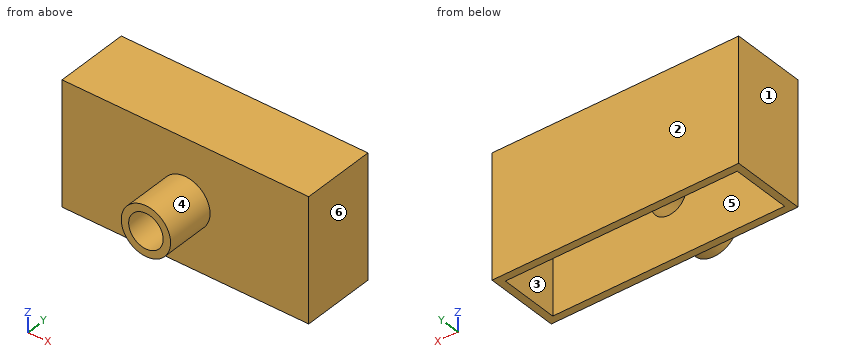
```python
from build123d import *

# Parameters (mm, degrees)
F0_W     = 254
F0_H     = 127
F1_DEPTH = 76.2
F2_W     = 25.4
F2_H     = 50.8
F4_T     = -7.62


with BuildPart() as f1:
    # F0 (on Front) → F1 (new body)
    with BuildSketch(Plane.XZ):
        Rectangle(F0_W, F0_H)
    extrude(amount=F1_DEPTH)

    # F2 (on Top) → F3 (revolve)
    with BuildSketch(Plane.XY):
        with Locations((12.7, -101.6)):
            Rectangle(F2_W, F2_H)
    revolve(axis=Axis((0, -101.6, 0), (0, 1, 0)))

    # F4
    f4_openings = [f1.faces().sort_by_distance(p)[0] for p in [
        (0, -127, 0),
        (0, -38.1, -63.5),
    ]]
    offset(amount=F4_T, openings=f4_openings, kind=Kind.INTERSECTION)


solid = f1.part
```
Source: CAD feature listing. Evaluate the final solid. Frame: model axes, mm. Face numbers are marked on the shaded views. A direction names the side the tool comes from. Coordinates: 2 decimals unless noted, no trailing zeros. Loops run counter-clockwise (first coordinate to the right, second up) from the corner with the lowest first, then second, coordinate; pieces in that order, holes last. Notation, with made-up numbers: (48.5, 84.25) -> (74.5, 84.25) arc R20 cw to (74.5, 122.25) -> close; hole circle Ø2 at (31, 20). An arc over 180 degrees is marked (long way). One line per item, written item: value. Start each with the question number.
Q1. Section query C-C, the plane y = -59. Return the cut outline in (x, z).
Q2. Section query D-D, the plane x = 75. Return the cut outline in (y, z).
Q3. Contact query for flat-ended pins moving along their axis: P1, Ø21.5, axis at x = 0, z = 0, coming from the -Y side; P2, Ø10, axis at x = -22, y = -28.5, coming from the -Z side. Output: stop coordinate, or through.
Q4. Section query A-A, the plane z = 48. Return the cut outline in (x, y), and give its area (3 significant figures).
Q5. Mould query, pull axis Y, two halves, no side actions, for the marked faces 1, 2 and 3. Classes: pulls with the +Y half, pulls with the -Y half, needs draft (parallel to the pull), parting line crosses it, or undercut.
Q6. Section query B-B, the plane x = 0. Return the cut outline in (y, z).
Q7. Set-up query: the marked faces 4, 5 and 6. Return all of +Z, -Z, +X, -X, +Y, -Y with unobstructed straight access to the full face (end or side cutting, diameter ignored); none if empty.
Q8. Line query: line 1 along Y through (x, z) = (79, 15.5); line 2 along X through (y, z) = (-107.5, 0); line 3 along X through (y, z) = (-36, 40.5). Output: solid intervals per line, ascending.
Results:
1. outline: (-127, -63.5) -> (-119.38, -63.5) -> (-119.38, 55.88) -> (119.38, 55.88) -> (119.38, -63.5) -> (127, -63.5) -> (127, 63.5) -> (-127, 63.5) -> close
2. outline: (-76.2, -63.5) -> (-68.58, -63.5) -> (-68.58, 55.88) -> (-7.62, 55.88) -> (-7.62, -63.5) -> (0, -63.5) -> (0, 63.5) -> (-76.2, 63.5) -> close
3. P1: y = -7.62
3. P2: z = 55.88
4. outline: (-127, -76.2) -> (127, -76.2) -> (127, 0) -> (-127, 0) -> close; hole (-119.38, -68.58) -> (119.38, -68.58) -> (119.38, -7.62) -> (-119.38, -7.62) -> close
4. area: 4,800 mm^2
5. face 1: needs draft
5. face 2: pulls with the +Y half
5. face 3: undercut
6. outline: (-127, -25.4) -> (-76.2, -25.4) -> (-76.2, -63.5) -> (-68.58, -63.5) -> (-68.58, -17.78) -> (-127, -17.78) -> close; (-127, 17.78) -> (-68.58, 17.78) -> (-68.58, 55.88) -> (-7.62, 55.88) -> (-7.62, -63.5) -> (0, -63.5) -> (0, 63.5) -> (-76.2, 63.5) -> (-76.2, 25.4) -> (-127, 25.4) -> close
7. face 4: -Y
7. face 5: -Z
7. face 6: +Z, -Z, +X, +Y, -Y
8. line 1: -76.2 to -68.58, -7.62 to 0
8. line 2: -25.4 to -17.78, 17.78 to 25.4
8. line 3: -127 to -119.38, 119.38 to 127
